The model under review builds one solid part; all positions refer to its coordinate system, in mm. Coordinates: 2 decimals unless noted, no trailing zeros. Write each loop counter-clockwise with the first axis right and the second up, starting at its lowest first coordinate (ties: lowest second). Pieces come first, ordered by that corner, then holes.
1) Add section B-B, the plane x = 14. State the section outline as (y, z) points, then the cut area to 3 significant figures.
2) For P1, Ø3, axis at x = 10.5, y = 12.5, coming from the -Z side; P2, Ø1, axis at x = -6.5, z = 1, coming from the +Y side, all flat-tipped, find the tip position at first contact; note any pin that passes through.
3) Add section C-C, the plane y = 25. State the section outline as (x, z) points.
4) Add section A-A, the plane z = 0.4. State the section outline as (x, y) points.
5) For line 1 (Y direction, x = 16.5, z = 0.5); line 2 (Y direction, x = 17, z = 0.9); line 3 (X direction, y = 25, z = 1.8), list the stretches that pass through material, from the lowest coordinate up.
from build123d import *

# Parameters (mm, degrees)
F1_DEPTH = 2
F2_R     = 5


with BuildPart() as f1:
    # F0 (on Top) → F1 (new body)
    with BuildSketch(Plane.XY):
        Polygon((30.310889, -17.5), (0, 35), (-30.310889, -17.5), align=None)
    extrude(amount=F1_DEPTH)

    # F2
    f2_edges = [f1.edges().sort_by_distance(p)[0] for p in [
        (0, 35, 1),
        (-30.310889, -17.5, 1),
        (30.310889, -17.5, 1),
    ]]
    fillet(f2_edges, radius=F2_R)


solid = f1.part
Geometry results:
1. outline: (-17.5, 0) - (10.75, 0) - (10.75, 2) - (-17.5, 2) - close
1. area: 56.5 mm2
2. P1: stops at z = 0
2. P2: stops at y = 24.61
3. outline: (-5.77, 0) - (5.77, 0) - (5.77, 2) - (-5.77, 2) - close
4. outline: (-25.98, -10) arc R5 ccw to (-21.65, -17.5) - (21.65, -17.5) arc R5 ccw to (25.98, -10) - (4.33, 27.5) arc R5 ccw to (-4.33, 27.5) - close
5. line 1: y = -17.5 to 6.42
5. line 2: y = -17.5 to 5.56
5. line 3: x = -5.77 to 5.77
